```python
from build123d import *

# Parameters (mm, degrees)
SKETCH1_W                                       = 15
SKETCH1_H                                       = 47
BOSS_EXTRUDE1_DEPTH                             = 42.5
SKETCH2_W                                       = 30
SKETCH2_H                                       = 30
CUT_EXTRUDE1_DEPTH                              = 16
SKETCH3_R                                       = 2.75
CUT_EXTRUDE2_DEPTH                              = 15
CUT_EXTRUDE3_REACH                              = 49
SKETCH4_R                                       = 3.25
SKETCH5_R                                       = 2.75
CUT_EXTRUDE4_DEPTH                              = 28.5
CUT_EXTRUDE6_START                              = -7.2
SKETCH6_R                                       = 6.3
CUT_EXTRUDE6_DEPTH                              = 15
CSK_FOR_M6_FLAT_HEAD_MACHINE_SCREW1_D           = 6.6
CSK_FOR_M6_FLAT_HEAD_MACHINE_SCREW1_CSINK_D     = 12.6
CSK_FOR_M6_FLAT_HEAD_MACHINE_SCREW1_CSINK_ANGLE = 90
SKETCH10_W                                      = 8.2
SKETCH10_H                                      = 4.2
CUT_EXTRUDE7_DEPTH                              = 12


with BuildPart() as part:
    # Sketch1 → Boss-Extrude1 (new body)
    with BuildSketch(Plane.XY):
        with Locations((7.5, 23.5)):
            Rectangle(SKETCH1_W, SKETCH1_H)
    extrude(amount=BOSS_EXTRUDE1_DEPTH)

    # Sketch2 → Cut-Extrude1 (cut, through all)
    with BuildSketch(Plane.ZY):
        with Locations((15, 15)):
            Rectangle(SKETCH2_W, SKETCH2_H)
    extrude(amount=-CUT_EXTRUDE1_DEPTH, mode=Mode.SUBTRACT)

    # Sketch3 → Cut-Extrude2 (cut)
    with BuildSketch(Plane.XY.offset(42.5)):
        with Locations((7.5, 15)):
            Circle(SKETCH3_R)
        with Locations((7.5, 40)):
            Circle(SKETCH3_R)
    extrude(amount=-CUT_EXTRUDE2_DEPTH, mode=Mode.SUBTRACT)

    # Sketch4 → Cut-Extrude3 (cut, up to next)
    with BuildSketch(Plane(origin=(0, 47, 0), x_dir=(1, 0, 0), z_dir=(0, 1, 0)), mode=Mode.PRIVATE) as cut_extrude3_sk1:
        with Locations((7.5, -15)):
            Circle(SKETCH4_R)
    cut_extrude3_tool1 = extrude(cut_extrude3_sk1.sketch, amount=-CUT_EXTRUDE3_REACH, mode=Mode.PRIVATE) & part.part
    add(cut_extrude3_tool1.solids().sort_by_distance((7.5, 47, 15))[0], mode=Mode.SUBTRACT)

    # Sketch5 → Cut-Extrude4 (cut, through all)
    with BuildSketch(Plane.XY.offset(27.5)):
        with Locations((7.5, 40)):
            Circle(SKETCH5_R)
    extrude(amount=-CUT_EXTRUDE4_DEPTH, mode=Mode.SUBTRACT)

    # Sketch6 → Cut-Extrude6 (cut)
    with BuildSketch(Plane.XZ.offset(-30).offset(CUT_EXTRUDE6_START)):
        with Locations((7.5, 15)):
            Circle(SKETCH6_R)
    extrude(amount=-CUT_EXTRUDE6_DEPTH, mode=Mode.SUBTRACT)

    # CSK for M6 Flat Head Machine Screw1 (through all)
    with Locations(Plane(origin=(0, 37.2, 0), x_dir=(1, 0, 0), z_dir=(0, 1, 0))):
        with Locations((7.5, -15)):
            CounterSinkHole(CSK_FOR_M6_FLAT_HEAD_MACHINE_SCREW1_D / 2, CSK_FOR_M6_FLAT_HEAD_MACHINE_SCREW1_CSINK_D / 2, counter_sink_angle=CSK_FOR_M6_FLAT_HEAD_MACHINE_SCREW1_CSINK_ANGLE)

    # Sketch10 → Cut-Extrude7 (cut)
    with BuildSketch(Plane(origin=(0, 47, 0), x_dir=(1, 0, 0), z_dir=(0, 1, 0))):
        with Locations((7.5, -36.4)):
            Rectangle(SKETCH10_W, SKETCH10_H)
        with Locations((7.5, -27.7)):
            Rectangle(SKETCH10_W, SKETCH10_H)
    extrude(amount=-CUT_EXTRUDE7_DEPTH, mode=Mode.SUBTRACT)


solid = part.part
```
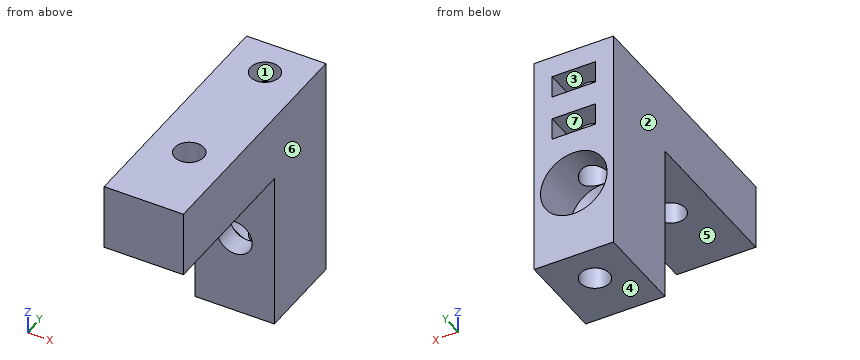
Part model, mm, in its own coordinate system. Face numbers are marked on the shaded views. A direction names the side the tool comes from. Round coordinates to 2 decimals unless told otherwise and drop trailing zeros. Loops run counter-clockwise (first coordinate to the right, second up) from the corner with the lowest first, then second, coordinate; pieces in that order, holes last. Notation, with made-up numbers: (18.25, 14.25) -> (68.25, 14.25) arc R19 ccw to (68.25, 18.25) -> close; hole circle Ø4 at (60, -4). An arc over 180 degrees is marked (long way). Use CSV: the item, a comma, the result in double quotes. Start each with the question number.
1) Which spindle directions (+Z, -Z, +X, -X, +Y, -Y) get a long thin tool onto all of the face, cutting with end or side? Do the marked faces 5, 6 and 7. Say none if no direction does.
2) Pull direction X, two halves, no side cores. Call the marked faces 1, 2, 3 and 4: +X half, -X half, draft (parallel to the pull), parting line (faces both ways), or undercut.
3) Cut at A-A, the plane z = 15. Write the cut outline in (x, y).
4) Drop flat-ended pins along their axis: P1, Ø3.5, axis at x = 8.5, z = 27.5, coming from the +Y side; P2, Ø3, axis at x = 13, y = 11.5, coming from the -Z side; P3, Ø3.5, axis at x = 7.5, y = 40, coming from the -Z side; P4, Ø1, axis at x = 9, z = 6.5, coming from the -Y side. Give the stop position or say it passes through.
5) Cut at B-B, the plane y = 15. Write the cut outline in (x, z), plus the area to 3 significant figures.
6) Cut at C-C, the plane x = 7.5. Give the number of separate pieces and of enclosed holes in the cut face, plus the area to 3 significant figures.
7) Wall check: L1, parallel to Y at x = 7.5, z = 39; L2, parallel to Z at x = 7.5, y = 32.55; L3, parallel to X at y = 40, z = 22. Give the ranges that are in metal, low to high. Write a range as [from, to].
8) Cut at D-D, the plane y = 40. Write the cut outline in (x, z), plus the area to 3 significant figures.
Determined:
1,face 5,"-Z, +X, -X, -Y"
1,face 6,"+Z, -Z, +X, +Y, -Y"
1,face 7,"+Y"
2,face 1,"undercut"
2,face 2,"-X half"
2,face 3,"undercut"
2,face 4,"draft"
3,outline,"(0, 30) -> (4.2, 30) -> (4.2, 34.2) -> (1.2, 37.2) -> (1.2, 47) -> (0, 47) -> close; (10.8, 30) -> (15, 30) -> (15, 47) -> (13.8, 47) -> (13.8, 37.2) -> (10.8, 34.2) -> close"
4,P1,"stops at y = 35"
4,P2,"stops at z = 30"
4,P3,"passes through"
4,P4,"stops at y = 30"
5,outline,"(0, 30) -> (4.75, 30) -> (4.75, 42.5) -> (0, 42.5) -> close; (10.25, 30) -> (15, 30) -> (15, 42.5) -> (10.25, 42.5) -> close"
5,area,"119 mm2"
6,separate pieces,"7"
6,enclosed holes,"0"
6,area,"630 mm2"
7,L1,"y = [0, 12.25], [17.75, 37.25], [42.75, 47]"
7,L2,"z = [0, 11.7], [18.3, 42.5]"
7,L3,"x = [0, 4.75], [10.25, 15]"
8,outline,"(0, 0) -> (4.75, 0) -> (4.75, 9.33) arc R6.3 cw to (4.75, 20.67) -> (4.75, 25.6) -> (3.4, 25.6) -> (3.4, 29.8) -> (4.75, 29.8) -> (4.75, 34.3) -> (3.4, 34.3) -> (3.4, 38.5) -> (4.75, 38.5) -> (4.75, 42.5) -> (0, 42.5) -> close; (10.25, 0) -> (15, 0) -> (15, 42.5) -> (10.25, 42.5) -> (10.25, 38.5) -> (11.6, 38.5) -> (11.6, 34.3) -> (10.25, 34.3) -> (10.25, 29.8) -> (11.6, 29.8) -> (11.6, 25.6) -> (10.25, 25.6) -> (10.25, 20.67) arc R6.3 cw to (10.25, 9.33) -> close"
8,area,"323 mm2"
